Read the model definition and answer for the solid it produces. Units are mm, in the model's axes. A direction names the side the tool comes from. Coordinates: 2 decimals unless noted, no trailing zeros. Loops run counter-clockwise (first coordinate to the right, second up) from the corner with the lowest first, then second, coordinate; pieces in that order, holes last. Notation, with made-up numbers: (85.25, -14.5) -> (117.25, -14.5) arc R23 cw to (117.25, 15.5) -> close; hole circle Ø3 at (88.5, 85.25). An arc over 180 degrees is marked (long way). Answer in a Markdown table with one row per item.
```python
from build123d import *

# Parameters (mm, degrees)
ESQUISSE1_W        = 50
ESQUISSE1_H        = 80
BOSS_EXTRU_1_DEPTH = 10


with BuildPart() as part:
    # Esquisse1 → Boss.-Extru.1 (new body)
    with BuildSketch(Plane.XY):
        with Locations((3.064709519, 0)):
            Rectangle(ESQUISSE1_W, ESQUISSE1_H)
        with BuildLine():
            Line((-13.904077664, -30), (-13.904077664, 30))
            ThreePointArc((-13.904077664, 30), (-11.904077664, 32), (-9.904077664, 30))
            Line((-9.904077664, 30), (-9.904077664, -30))
            ThreePointArc((-9.904077664, -30), (-11.904077664, -32), (-13.904077664, -30))
        make_face(mode=Mode.SUBTRACT)
        Polygon((-4.435290481, -30), (-4.435290481, 0), (-4.435290481, 30), (10.564709519, 30), (10.564709519, 0), (10.564709519, -30), align=None, mode=Mode.SUBTRACT)
        with BuildLine():
            Line((16.033496703, -30), (16.033496703, 30))
            ThreePointArc((16.033496703, 30), (18.033496703, 32), (20.033496703, 30))
            Line((20.033496703, 30), (20.033496703, -30))
            ThreePointArc((20.033496703, -30), (18.033496703, -32), (16.033496703, -30))
        make_face(mode=Mode.SUBTRACT)
    extrude(amount=BOSS_EXTRU_1_DEPTH)


solid = part.part
```
1. A tool of negligible diameter and unlimited length cuts with its end or side. For faces 4 (the flat face through (16.033, 0, 5)), 5 (the flat face through (28.065, -1, 5)), from which of +Z, -Z, +X, -X, +Y, -Y can it reach the whole face along a straight path? Write none if from no direction.
A:
| item | result |
|---|---|
| face 4 | +Z, -Z |
| face 5 | +Z, -Z, +X, +Y, -Y |
2. Find the intervals of material crossed by probe 1 along X at (y, z) = (-7, 9.75); probe 2 along Y at (x, z) = (8, 9.25); probe 3 along Y at (x, z) = (19, 3.25), in increasing order.
A:
| item | result |
|---|---|
| probe 1 | x = -21.94 to -13.9, -9.9 to -4.44, 10.56 to 16.03, 20.03 to 28.06 |
| probe 2 | y = -40 to -30, 30 to 40 |
| probe 3 | y = -40 to -31.75, 31.75 to 40 |
3. A cutting plane is placed at C-C on y = -12. Give the vertices of the cut face in (x, z).
A:
| item | result |
|---|---|
| outline | (-21.94, 0) -> (-13.9, 0) -> (-13.9, 10) -> (-21.94, 10) -> close; (-9.9, 0) -> (-4.44, 0) -> (-4.44, 10) -> (-9.9, 10) -> close; (10.56, 0) -> (16.03, 0) -> (16.03, 10) -> (10.56, 10) -> close; (20.03, 0) -> (28.06, 0) -> (28.06, 10) -> (20.03, 10) -> close |
4. The mould has two halves that part along X. Classify faces 1 (the flat face through (-21.935, -1, 5)), 2 (the flat face through (3, 40, 5)), 3 (the flat face through (-13.904, 0, 5)): pulls with the +X half, pulls with the -X half, needs draft (parallel to the pull), parting line crosses it, or undercut.
A:
| item | result |
|---|---|
| face 1 | pulls with the -X half |
| face 2 | needs draft |
| face 3 | undercut |
5. A cutting plane is placed at A-A on z = 7.5. Give the vertices of the cut face in (x, y).
A:
| item | result |
|---|---|
| outline | (-21.94, -40) -> (28.06, -40) -> (28.06, 40) -> (-21.94, 40) -> close; hole (-13.9, -30) arc R2 ccw to (-9.9, -30) -> (-9.9, 30) arc R2 ccw to (-13.9, 30) -> close; hole (-4.44, -30) -> (10.56, -30) -> (10.56, 30) -> (-4.44, 30) -> close; hole (16.03, -30) arc R2 ccw to (20.03, -30) -> (20.03, 30) arc R2 ccw to (16.03, 30) -> close |
6. A cutting plane is placed at B-B on x = 1.5. Give the vertices of the cut face in (y, z), and give its area (3 significant figures).
A:
| item | result |
|---|---|
| outline | (-40, 0) -> (-30, 0) -> (-30, 10) -> (-40, 10) -> close; (30, 0) -> (40, 0) -> (40, 10) -> (30, 10) -> close |
| area | 200 mm2 |
7. Given pin 1 Ø1.5 at (x, y) = (22.5, -0.5) entering from -Z, flat-ended and moving along its own axis, determine where the tip first touches the part or whether it passes through.
A:
| item | result |
|---|---|
| pin 1 | stops at z = 0 |
